```python
from build123d import *


with BuildPart() as f4:
    # F4: sweep along a path in F0
    with BuildLine(Plane.XY) as f4_path:
        Line((5, 0), (35, 0))
        ThreePointArc((35, 0), (38.5355339059, 1.4644660941), (40, 5))
        Line((40, 5), (40, 25))
        ThreePointArc((40, 25), (38.5355339059, 28.5355339059), (35, 30))
        Line((35, 30), (5, 30))
        ThreePointArc((5, 30), (1.4644660941, 28.5355339059), (0, 25))
        Line((0, 25), (0, 5))
        ThreePointArc((0, 5), (1.4644660941, 1.4644660941), (5, 0))
    # F3 (on line) → F4 (sweep)
    with BuildSketch(Plane.YZ.offset(20)):
        Polygon((-2, 0), (0, 0), (0, 0.8), (-0.4, 0.8), (-1, 1.4), (-1.6, 0.8), (-2, 0.8), align=None)
    sweep(path=f4_path.line)


solid = f4.part
```
Geometry: final body of the model. Coordinates: model frame, mm. A direction names the side the tool comes from. Round coordinates to 2 decimals unless told otherwise and drop trailing zeros. Write each loop counter-clockwise with the first axis right and the second up, starting at its lowest first coordinate (ties: lowest second). Pieces come first, ordered by that corner, then holes.
Item 1: Set-up query: faces 1 (the face through (40, 29.9, 0.4)), 2 (the face through (1.5, 28.57, 0.41)), 3 (the face through (38.9, 1.02, 0.97)). Return all of +Z, -Z, +X, -X, +Y, -Y with unobstructed straight access to the full face (end or side cutting, diameter ignored); none if empty.
Item 2: Mould query, pull axis X, two halves, no side actions, for faces 4 (the face through (0.589, 0.685, 1.229)), 5 (the face through (39.411, 29.315, 1.229)), 6 (the face through (1.02, 1.1, 0.97)), 7 (the face through (38.57, 28.5, 0.41)). Classes: +X half, -X half, draft (parallel to the pull), parting line (faces both ways), or undercut.
Item 3: Section query B-B (y = 8.5). Return loops of the section in (x, z).
Item 4: Section query A-A (z = 0.45). Return loops of the section in (x, y), plus the area to 3 significant figures.
Item 5: Material intervals for L1, parallel to Y at x = 13, z = 0.1; L2, parallel to X at y = 22, z = 0.6; L3, parallel to X at y = 2.5, z = 0.25, sorted ascending.
Item 6: Pin query (flat end, axial travel): P1, Ø1.5, axis at x = 17.5, y = 2, coming from the -Z side. Return the tip coordinate at first contact, or that it passes through.
Item 7: Section query C-C (x = 12). Return loops of the section in (y, z), plus the area to 3 significant figures.
Completed:
1. face 1: +Z, -Z, +X, +Y
1. face 2: +Z, -Z
1. face 3: +Z
2. face 4: -X half
2. face 5: +X half
2. face 6: undercut
2. face 7: undercut
3. outline: (-2, 0) - (0, 0) - (0, 0.8) - (-0.4, 0.8) - (-1, 1.4) - (-1.6, 0.8) - (-2, 0.8) - close; (40, 0) - (42, 0) - (42, 0.8) - (41.6, 0.8) - (41, 1.4) - (40.4, 0.8) - (40, 0.8) - close
4. outline: (-2, 5) arc R7 ccw to (5, -2) - (35, -2) arc R7 ccw to (42, 5) - (42, 25) arc R7 ccw to (35, 32) - (5, 32) arc R7 ccw to (-2, 25) - close; hole (0, 5) arc R5 ccw to (5, 0) - (35, 0) arc R5 ccw to (40, 5) - (40, 25) arc R5 ccw to (35, 30) - (5, 30) arc R5 ccw to (0, 25) - close
4. area: 275 mm2
5. L1: y = -2 to 0, 30 to 32
5. L2: x = -2 to 0, 40 to 42
5. L3: x = -1.54 to 0.67, 39.33 to 41.54
6. P1: passes through
7. outline: (-2, 0) - (0, 0) - (0, 0.8) - (-0.4, 0.8) - (-1, 1.4) - (-1.6, 0.8) - (-2, 0.8) - close; (30, 0) - (32, 0) - (32, 0.8) - (31.6, 0.8) - (31, 1.4) - (30.4, 0.8) - (30, 0.8) - close
7. area: 3.92 mm2
